Here's how the part is built. I have some questions about the finished solid (model axes, mm). A direction names the side the tool comes from. Coordinates: 2 decimals unless noted, no trailing zeros. Loops run counter-clockwise (first coordinate to the right, second up) from the corner with the lowest first, then second, coordinate; pieces in that order, holes last.
```python
from build123d import *

# Parameters (mm, degrees)
F0_W      = 762
F0_H      = 990.6
F1_DEPTH  = 533.4
F2_W      = 177.8
F2_H      = 355.6
F3_DEPTH  = 495.3
F4_DEPTH  = 1188.72
F6_DEPTH  = 406.4
F8_DEPTH  = 406.4
F10_DEPTH = 533.4
F11_R     = 101.6
F12_DEPTH = 533.4
F14_DEPTH = 751.84
F16_DEPTH = 1084.58


with BuildPart() as f1:
    # F0 (on Right) → F1 (new body)
    with BuildSketch(Plane.YZ):
        Rectangle(F0_W, F0_H)
    extrude(amount=F1_DEPTH)

    # F2 (on face) → F3 (cut)
    with BuildSketch(Plane.XY.offset(495.3)):
        with Locations((88.9, -203.2)):
            Rectangle(F2_W, F2_H)
        with Locations((444.5, -203.2)):
            Rectangle(F2_W, F2_H)
    extrude(amount=-F3_DEPTH, mode=Mode.SUBTRACT)

    # F2 (on face) → F4 (cut)
    with BuildSketch(Plane.XY.offset(495.3)):
        with BuildLine():
            Line((355.6, -381), (355.6, -25.4))
            ThreePointArc((355.6, -25.4), (266.7, 63.5), (177.8, -25.4))
            Line((177.8, -25.4), (177.8, -381))
            Line((177.8, -381), (355.6, -381))
        make_face()
    extrude(amount=-F4_DEPTH, mode=Mode.SUBTRACT)

    # F5 (on face) → F6 (cut)
    with BuildSketch(Plane.XZ.offset(381)):
        with BuildLine():
            Line((533.4, -495.3), (533.4, -362.2072915536))
            ThreePointArc((533.4, -362.2072915536), (452.6800879623, -430.0887112407), (355.6, -471.3082194778))
            Line((355.6, -471.3082194778), (355.6, -495.3))
            Line((355.6, -495.3), (533.4, -495.3))
        make_face()
    extrude(amount=-F6_DEPTH, mode=Mode.SUBTRACT)

    # F7 (on face) → F8 (cut)
    with BuildSketch(Plane.XZ.offset(381)):
        with BuildLine():
            ThreePointArc((177.8, -471.3082194778), (80.7199120377, -430.0887112407), (0, -362.2072915536))
            Line((0, -362.2072915536), (0, -495.3))
            Line((0, -495.3), (177.8, -495.3))
            Line((177.8, -495.3), (177.8, -471.3082194778))
        make_face()
    extrude(amount=-F8_DEPTH, mode=Mode.SUBTRACT)

    # F9 (on face) → F10 (join)
    with BuildSketch(Plane(origin=(0, 381, 0), x_dir=(-1, 0, 0), z_dir=(0, 1, 0))):
        with BuildLine():
            ThreePointArc((-266.7, -139.7), (-123.0159020629, -80.1840979371), (-63.5, 63.5))
            ThreePointArc((-63.5, 63.5), (-410.3840979371, 207.1840979371), (-266.7, -139.7))
        make_face()
    extrude(amount=F10_DEPTH)

    # F11 (on face) → F12 (cut)
    with BuildSketch(Plane(origin=(0, 914.4, 0), x_dir=(-1, 0, 0), z_dir=(0, 1, 0))):
        with Locations((-266.7, 63.5)):
            Circle(F11_R)
    extrude(amount=-F12_DEPTH, mode=Mode.SUBTRACT)

    # F14 (cut): a face of the model
    f14_faces = [f1.faces().sort_by_distance(p)[0] for p in [
        (355.6, 0, -483.3041097389),
    ]]
    extrude(f14_faces, amount=-F14_DEPTH, mode=Mode.SUBTRACT)

    # F15 (on face) → F16 (cut)
    with BuildSketch(Plane.YZ.offset(533.4)):
        with BuildLine():
            ThreePointArc((152.4, -165.1), (174.7184632736, -218.9815367264), (228.6, -241.3))
            Line((228.6, -241.3), (228.6, -165.1))
            Line((228.6, -165.1), (152.4, -165.1))
        make_face()
        with BuildLine():
            ThreePointArc((152.4, 114.3), (-194.4840979371, 257.9840979371), (-50.8, -88.9))
            ThreePointArc((-50.8, -88.9), (92.8840979371, -29.3840979371), (152.4, 114.3))
        make_face()
        with BuildLine():
            Line((228.6, -165.1), (228.6, -241.3))
            ThreePointArc((228.6, -241.3), (282.4815367264, -218.9815367264), (304.8, -165.1))
            ThreePointArc((304.8, -165.1), (228.6, -88.9), (152.4, -165.1))
            Line((152.4, -165.1), (228.6, -165.1))
        make_face()
    extrude(amount=-F16_DEPTH, mode=Mode.SUBTRACT)


solid = f1.part
```
1. I want a section at A-A (z = -165.1). Please give me the cut outline in (x, y).
2. For pin 1 (10 mm diameter, centred on x = 197, z = -372.5, fed in from +Y); pin 2 (10 mm diameter, centred on x = 170, z = 48, fed in from -Y); pin 3 (4 mm diameter, centred on y = 647.5, z = 88, fed in from +X), each with a flat end and sliding along its axis, tell me the tip position at first contact or that it passes through.
3. I want a section at D-D (z = 351). Please give me the cut outline in (x, y).
4. We'd pull the mould along Y, two halves only. Please class faces 1 (the cylindrical face through (270.434, 231.95, -88.974)), 2 (the flat face through (88, -25.4, 407)), 3 (the flat face through (144, 381, -117)), 4 (the flat face through (0, 79, -103)): +Y half, -Y half, draft (parallel to the pull), parting line (faces both ways), or undercut.
5. I want a section at B-B (y = -50.8). Please give me the cut outline in (x, z).
6. I want a section at C-C (x = 270). Please give me the cut outline in (y, z).
7. On a 3-axis mill with a long thin cutter (end or side, diameter ignored), from which of +Z, -Z, +X, -X, +Y, -Y can I reach the whole of each face in a straight line? I mean faces 5 (the cylindrical face through (81.98, -180.64, -430.86)), 6 (the cylindrical face through (453.94, -180.64, -429.31)), 7 (the flat face through (268, 381, 65)), 8 (the flat face through (88, -299, 0)). Say none if no direction works.
8. I need wall thicknesses on line 1 along Z through (x, y) = (209, 63); line 2 along Z through (x, y) = (266.7, 667); line 3 along Y through (x, z) = (154, -165). Which ranges of each line are inside material? Lowest first, please.
Response values:
1. outline: (0, -381) - (177.8, -381) - (177.8, -25.4) arc R88.9 cw to (355.6, -25.4) - (355.6, -381) - (533.4, -381) - (533.4, 152.4) - (0, 152.4) - close; (0, 304.8) - (533.4, 304.8) - (533.4, 381) - (0, 381) - close
2. pin 1: stops at y = 381
2. pin 2: stops at y = 139.48
2. pin 3: stops at x = 468.65
3. outline: (0, -25.4) - (177.8, -25.4) arc R88.9 cw to (355.6, -25.4) - (533.4, -25.4) - (533.4, 381) - (0, 381) - close
4. face 1: undercut
4. face 2: -Y half
4. face 3: +Y half
4. face 4: draft
5. outline: (0, -362.21) arc R355.6 ccw to (177.8, -471.31) - (177.8, -88.9) - (0, -88.9) - close; (355.6, -471.31) arc R355.6 ccw to (533.4, -362.21) - (533.4, -88.9) - (355.6, -88.9) - close
6. outline: (63.44, -495.3) - (381, -495.3) - (381, -139.67) - (914.4, -139.67) - (914.4, -38.05) - (381, -38.05) - (381, 165.05) - (914.4, 165.05) - (914.4, 266.67) - (381, 266.67) - (381, 495.3) - (63.44, 495.3) - (63.44, 282.35) arc R203.2 cw to (63.44, -53.75) - close; hole circle Ø152.4 at (228.6, -165.1)
7. face 5: -Z, -X, -Y
7. face 6: -Z, +X, -Y
7. face 7: +Y
7. face 8: +Z, +X, -X, -Y
8. line 1: z = -495.3 to -54.04, 282.64 to 495.3
8. line 2: z = -139.7 to -38.1, 165.1 to 266.7
8. line 3: y = -381 to 152.4, 304.8 to 381
